Design review of the part built by this model. Coordinates are the model's own, in mm. A direction names the side the tool comes from. Coordinates: 2 decimals unless noted, no trailing zeros. Loops run counter-clockwise (first coordinate to the right, second up) from the corner with the lowest first, then second, coordinate; pieces in that order, holes last. Notation, with made-up numbers: (73, 47.25) -> (104, 47.25) arc R11 ccw to (104, 53.25) -> close; hole circle Ø1 at (85.5, 55). An arc over 180 degrees is marked (long way). Answer as a JSON object with one key per item and string values.
```python
from build123d import *

# Parameters (mm, degrees)
F1_DEPTH = 90
F2_DEPTH = 60
F4_DEPTH = 60.001


with BuildPart() as f1:
    # F0 (on Front) → F1 (new body)
    with BuildSketch(Plane.XZ):
        with BuildLine():
            Line((0, 0), (-20, 0))
            Line((-20, 0), (-20, -60))
            Line((-20, -60), (40, -60))
            Line((40, -60), (40, -40))
            ThreePointArc((40, -40), (11.715729, -28.284271), (0, 0))
        make_face()
        with BuildLine():
            Line((40, 0), (0, 0))
            ThreePointArc((0, 0), (11.715729, -28.284271), (40, -40))
            Line((40, -40), (40, 0))
        make_face()
    extrude(amount=-F1_DEPTH)

    # F0 (on Front) → F2 (cut)
    with BuildSketch(Plane.XZ):
        with BuildLine():
            Line((40, 0), (0, 0))
            ThreePointArc((0, 0), (11.715729, -28.284271), (40, -40))
            Line((40, -40), (40, 0))
        make_face()
    extrude(amount=-F2_DEPTH, mode=Mode.SUBTRACT)

    # F3 (on face) → F4 (cut, through all)
    with BuildSketch(Plane.XY):
        with BuildLine():
            Line((32, 90), (-12, 90))
            ThreePointArc((-12, 90), (10, 68), (32, 90))
        make_face()
    extrude(amount=-F4_DEPTH, mode=Mode.SUBTRACT)


solid = f1.part
```
1) Clearance check with flat-ended pins moving along their axes: pin 1 Ø12 at (x, z) = (17.5, -18) entering from -Y; pin 2 Ø6 at (x, z) = (5.5, -39.5) entering from +Y; pin 3 Ø2 at (y, z) = (30.5, -17) entering from +X. State where each tip first meets the part, or that it passes through.
Completed:
{"pin 1": "y = 60", "pin 2": "y = 69.32", "pin 3": "x = 4.28"}
2) Wall thickness on probe 1 along Y at (x, z) = (11, -25); probe 2 along Y at (x, z) = (11, -30.5); probe 3 along Z at (x, y) = (12.5, 11): over which ranges is each line inside the solid? List them lowest first.
Completed:
{"probe 1": "60 to 68.02", "probe 2": "0 to 68.02", "probe 3": "-60 to -29.05"}
3) Add section C-C, the plane x = 28. Give the boundary of the cut face in (y, z), and give its area (3 significant figures).
Completed:
{"outline": "(0, -60) -> (77.35, -60) -> (77.35, 0) -> (60, 0) -> (60, -38.16) -> (0, -38.16) -> close", "area": "2,350 mm²"}
4) For faces 5 (the flat face through (24, 60, -15)), 6 (the flat face through (36, 90, -30)), list the 3-axis set-ups (+Z, -Z, +X, -X, +Y, -Y) from which the entire face can be reached by the end or side of a thin tool; tool diameter is ignored.
Completed:
{"face 5": "+Z, +X, -Y", "face 6": "+Z, -Z, +X, -X, +Y"}
5) The part is to be moulded in two halves that separate along X. For faces 1 (the flat face through (-20, 44, -30)), 2 (the flat face through (40, 54, -44)), 3 (the cylindrical face through (10, 68, -30)), 4 (the flat face through (-16, 90, -30)), say which applies: pulls with the +X half, pulls with the -X half, needs draft (parallel to the pull), parting line crosses it, or undercut.
Completed:
{"face 1": "pulls with the -X half", "face 2": "pulls with the +X half", "face 3": "undercut", "face 4": "needs draft"}
6) Add section D-D, the plane y = 47. Give the boundary of the cut face in (x, z).
Completed:
{"outline": "(-20, -60) -> (40, -60) -> (40, -40) arc R40 cw to (0, 0) -> (-20, 0) -> close"}
7) Add section B-B, the plane z = -36. Give the boundary of the cut face in (x, y), and give its area (3 significant figures).
Completed:
{"outline": "(-20, 0) -> (22.56, 0) -> (22.56, 60) -> (40, 60) -> (40, 90) -> (32, 90) arc R22 cw to (-12, 90) -> (-20, 90) -> close", "area": "3,590 mm²"}
8) Add section A-A, the plane y = 73. Give the boundary of the cut face in (x, z), and give its area (3 significant figures).
Completed:
{"outline": "(-20, -60) -> (-3.96, -60) -> (-3.96, 0) -> (-20, 0) -> close; (23.96, -60) -> (40, -60) -> (40, 0) -> (23.96, 0) -> close", "area": "1,920 mm²"}
